from build123d import *

# Parameters (mm, degrees)
SKETCH274_AS_DRAWN_R                 = 3
EXTRUDE077_DEPTH                     = 1
EXTRUDE077_ONTO_SKETCH274_ROLL_ANGLE = 90
EXTRUDE076_DEPTH                     = 1
EXTRUDE076_ONTO_SKETCH273_ROLL_ANGLE = 90


with BuildPart() as extrude077:
    # Sketch274 as drawn → Extrude077 (new)
    with BuildSketch(Plane.XY):
        with Locations((2, 8)):
            Circle(SKETCH274_AS_DRAWN_R)
    extrude(amount=-EXTRUDE077_DEPTH)


with BuildPart() as extrude077_1:
    # Extrude077 onto Sketch274 roll: moved
    add(extrude077.part.rotate(Axis((0, 0, 0), (1, 0, 0)), EXTRUDE077_ONTO_SKETCH274_ROLL_ANGLE))


with BuildPart() as extrude077_2:
    # Extrude077 onto Sketch274 placement: moved
    add(extrude077_1.part.moved(Location((0, -1, -0.5))))


with BuildPart() as cut046:
    # Sketch273 as drawn → Extrude076 (new)
    with BuildSketch(Plane.XY):
        with BuildLine():
            ThreePointArc((7, 8), (0.418861, 12.743416), (-1.999999, 5))
            Line((-1.999999, 5), (0, 1.5))
            Line((0, 1.5), (7, 1.5))
            Line((7, 8), (7, 1.5))
        make_face()
    extrude(amount=-EXTRUDE076_DEPTH)


with BuildPart() as cut046_1:
    # Extrude076 onto Sketch273 roll: moved
    add(cut046.part.rotate(Axis((0, 0, 0), (1, 0, 0)), EXTRUDE076_ONTO_SKETCH273_ROLL_ANGLE))


with BuildPart() as cut046_2:
    # Extrude076 onto Sketch273 placement: moved
    add(cut046_1.part.moved(Location((0, -1, -0.5))))

    # Cut046: cut Extrude077
    add(extrude077_2.part, mode=Mode.SUBTRACT)


solid = cut046_2.part
Read the model definition and answer for the solid it produces. Units are mm, in the model's axes. Give positions to 0.01 mm unless a question says otherwise; leave off trailing zeros. Loops run counter-clockwise (first coordinate to the right, second up) from the corner with the lowest first, then second, coordinate; pieces in that order, holes last. Notation, with made-up numbers: M 9,-25 L 54,-25 A20 ccw 54,-16 Z; hole C 16,65 d9. An arc over 180 degrees is marked long. Write each question's results on one line, items separated by ' | '.
1. Straight lines are drawn through the part: line 1 (Z direction, x = 2, y = -0.7); line 2 (X direction, y = -0.9, z = 8); line 3 (Z direction, x = 4.75, y = -0.55). For each, find the intervals that lie inside material, in ascending order. Write a range as [from, to].
Values:
line 1: z = [1, 4.5], [10.5, 12.5] | line 2: x = [-2.97, -0.96], [4.96, 6.97] | line 3: z = [1, 6.3], [8.7, 11.68]
2. Section A-A on x = 2 is taken. Give the vertices of the cut face in (y, z).
Values:
outline: M -1,1 L 0,1 L 0,4.5 L -1,4.5 Z; M -1,10.5 L 0,10.5 L 0,12.5 L -1,12.5 Z
3. Section B-B on z = 5 is taken. Give the vertices of the cut face in (x, y).
Values:
outline: M -2.33,-1 L 0.34,-1 L 0.34,0 L -2.33,0 Z; M 3.66,-1 L 7,-1 L 7,0 L 3.66,0 Z
4. The mould has two halves that part along Z. Classify faces 1 (the face through (2, -1, 4)), 2 (the face through (-1.01, -0.51, 2.77)), 3 (the face through (4.77, -0.51, 6.35)): pulls with the +Z half, pulls with the -Z half, needs draft (parallel to the pull), parting line crosses it, or undercut.
Values:
face 1: needs draft | face 2: pulls with the -Z half | face 3: undercut
5. Section C-C on y = -0.35 is taken. Give the vertices of the cut face in (x, z).
Values:
outline: M -2,4.5 L 0,1 L 7,1 L 7,7.5 A5 ccw long Z; hole C 2,7.5 d6
